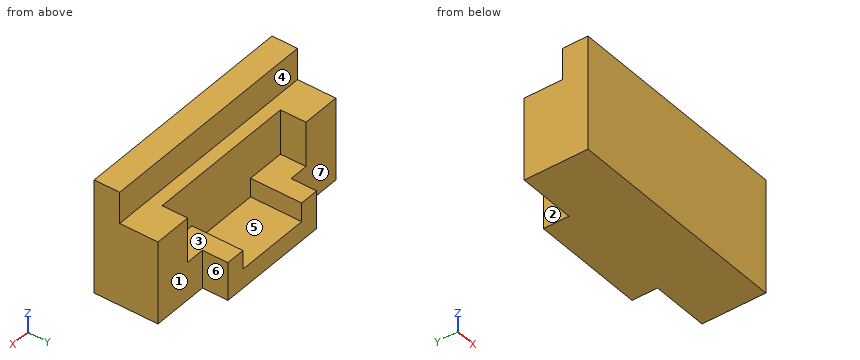
```python
from build123d import *

# Parameters (mm, degrees)
BOSS_EXTRUDE1_DEPTH = 57.15
BOSS_EXTRUDE2_DEPTH = 12.7
CUT_EXTRUDE1_DEPTH  = 25.4


with BuildPart() as part:
    # Sketch1 → Boss-Extrude1 (new, symmetric)
    with BuildSketch(Plane(origin=(0, 0, 0), x_dir=(0, 0, -1), z_dir=(1, 0, 0))):
        Polygon((-28.575, 0), (28.575, 0), (28.575, 31.75), (-12.827, 31.75), (-12.827, 12.7), (-28.575, 12.7), align=None)
    extrude(amount=BOSS_EXTRUDE1_DEPTH, both=True)

    # Sketch2 → Boss-Extrude2 (add)
    with BuildSketch(Plane(origin=(0, 31.75, 0), x_dir=(1, 0, 0), z_dir=(0, 1, 0))):
        Polygon((-28.448, 28.575), (28.575, 28.575), (28.575, 9.525), (18.923, 9.525), (18.923, 18.923), (-18.796, 18.923), (-18.796, 9.525), (-28.448, 9.525), align=None)
    extrude(amount=BOSS_EXTRUDE2_DEPTH)

    # Sketch3 → Cut-Extrude1 (cut)
    with BuildSketch(Plane(origin=(0, 44.45, 0), x_dir=(1, 0, 0), z_dir=(0, 1, 0))):
        Polygon((-18.796, 9.525), (-18.796, 18.923), (18.923, 18.923), (18.923, 9.525), (38.1, 9.525), (38.1, -12.827), (-37.973, -12.827), (-37.973, 9.525), align=None)
    extrude(amount=-CUT_EXTRUDE1_DEPTH, mode=Mode.SUBTRACT)


solid = part.part
```
CAD build for the part. Positions are in the model's coordinates, mm. Face numbers are marked on the shaded views. A direction names the side the tool comes from. Give positions to 0.01 mm unless a question says otherwise; leave off trailing zeros. Write each loop counter-clockwise with the first axis right and the second up, starting at its lowest first coordinate (ties: lowest second). Pieces come first, ordered by that corner, then holes. Notation, with made-up numbers: (-9.75, 36.25) -> (40.25, 36.25) arc R14 cw to (40.25, 54.25) -> close; hole circle Ø11 at (-15.75, 51). An arc over 180 degrees is marked (long way). Write each question's results on one line, items separated by ' | '.
1. Cut at B-B, the plane y = 38. Write the cut outline in (x, z) (3 decimals), then the cut area to 3 significant figures.
Geometry check:
outline: (-28.448, -28.575) -> (28.575, -28.575) -> (28.575, -9.525) -> (18.923, -9.525) -> (18.923, -18.923) -> (-18.796, -18.923) -> (-18.796, -9.525) -> (-28.448, -9.525) -> close | area: 732 mm²
2. Cut at D-D, the plane y = 22.5. Write the cut outline in (x, z) (3 decimals).
Geometry check:
outline: (-57.15, -28.575) -> (57.15, -28.575) -> (57.15, 12.827) -> (38.1, 12.827) -> (38.1, -9.525) -> (18.923, -9.525) -> (18.923, -18.923) -> (-18.796, -18.923) -> (-18.796, -9.525) -> (-37.973, -9.525) -> (-37.973, 12.827) -> (-57.15, 12.827) -> close
3. Wall check: probe 1 along X at (y, z) = (26, -2); probe 2 along X at (y, z) = (39, -12.5) (3 decimals); probe 3 along Y at (x, z) = (30, 3). Give the ranges that are in metal, low to high. Write a range as [from, to].
Geometry check:
probe 1: [-57.15, -37.97], [38.1, 57.15] | probe 2: [-28.448, -18.796], [18.923, 28.575] | probe 3: [0, 19.05]
4. Which spindle directions (+Z, -Z, +X, -X, +Y, -Y) get a long thin tool onto all of the face, cutting with end or side? Do the marked faces 1, 2, 3 and 4. Say none if no direction does.
Geometry check:
face 1: +Z, -Z, +X, +Y | face 2: +Z, -Z, -X, +Y | face 3: +Z, +Y | face 4: +Z, +X, -X, +Y
5. Cut at A-A, the plane x = -30.5. Write the cut outline in (y, z) (3 decimals).
Geometry check:
outline: (0, -28.575) -> (31.75, -28.575) -> (31.75, -9.525) -> (19.05, -9.525) -> (19.05, 12.827) -> (12.7, 12.827) -> (12.7, 28.575) -> (0, 28.575) -> close
6. Cut at C-C, the plane z = -11.5. Write the cut outline in (x, y) (3 decimals), then the cut area to 3 significant figures.
Geometry check:
outline: (-57.15, 0) -> (57.15, 0) -> (57.15, 31.75) -> (28.575, 31.75) -> (28.575, 44.45) -> (18.923, 44.45) -> (18.923, 19.05) -> (-18.796, 19.05) -> (-18.796, 44.45) -> (-28.448, 44.45) -> (-28.448, 31.75) -> (-57.15, 31.75) -> close | area: 3,400 mm²
7. Two-plate mould, pull along X, no slides. Class the marked faces 5, 6 and 7: pulls with the +X half, pulls with the -X half, needs draft (parallel to the pull), parting line crosses it, or undercut.
Geometry check:
face 5: undercut | face 6: pulls with the +X half | face 7: needs draft
8. Drop flat-ended pins along their axis: P1, Ø8.5, axis at x = -43, z = -10, coming from the +Y side; P2, Ø21, axis at x = 32, y = 31.5, coming from the +Z side; P3, Ø10, axis at x = 17.5, z = 20.5, coming from the +Y side. Give the stop position or say it passes through.
Geometry check:
P1: y = 31.75 | P2: z = 12.83 | P3: y = 12.7
